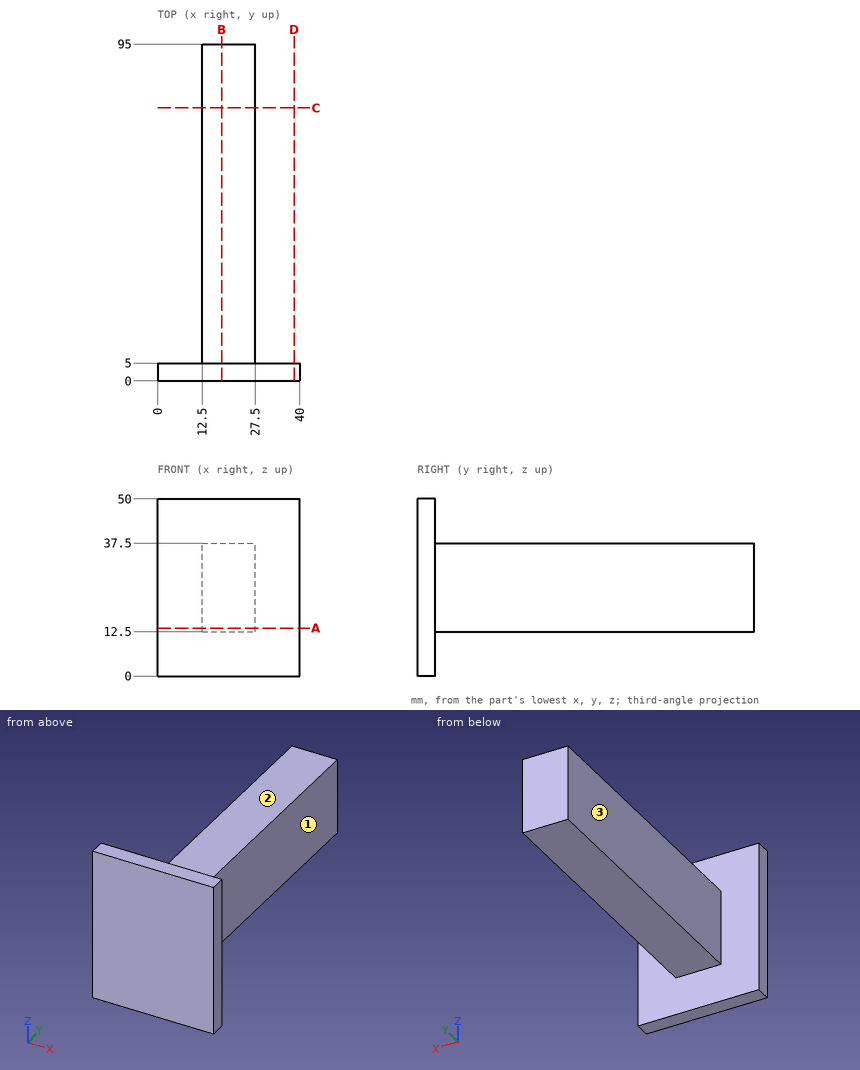
Study the drawing (mm; zero at the part's minimum x, y, z) and answer. A direction names the side the tool comes from. Give positions to 0.01 mm unless a question says otherwise; leave off trailing zeros. Write each loop counter-clockwise with the first axis right and the second up, starting at its lowest first coordinate (ties: lowest second). Pieces come first, ordered by that corner, then holes. Notation, with made-up numbers: (-22, 77) - (-15, 77) arc R11 ccw to (-15, 83) - close; hole circle Ø11 at (80, 68). An arc over 180 degrees is marked (long way). Use a Markdown table: item, result.
1. Section C-C on y = 77 is taken. Write down the section's boundary in (x, z), plus the area to 3 significant figures.
Values follow:
| item | result |
|---|---|
| outline | (12.5, 12.5) - (27.5, 12.5) - (27.5, 37.5) - (12.5, 37.5) - close |
| area | 375 mm² |
2. Section A-A on z = 13.5 is taken. Write down the section's boundary in (x, y), plus the area to 3 significant figures.
Values follow:
| item | result |
|---|---|
| outline | (0, 0) - (40, 0) - (40, 5) - (27.5, 5) - (27.5, 95) - (12.5, 95) - (12.5, 5) - (0, 5) - close |
| area | 1,550 mm² |
3. Each of these flat-tipped pins is pushed along its axis until it touches: P1, Ø12, axis at x = 21.5, y = 48, coming from the +Z side; P2, Ø6, axis at x = 24.5, y = 63.5, coming from the -Z side; P3, Ø2, axis at y = 32, z = 18.5, coming from the -X side. Where does it stop, or does it pass through?
Values follow:
| item | result |
|---|---|
| P1 | stops at z = 37.5 |
| P2 | stops at z = 12.5 |
| P3 | stops at x = 12.5 |
4. A tool of negligible diameter and unlimited length cuts with its end or side. For the marked faces 1, 2 and 3, from which of +Z, -Z, +X, -X, +Y, -Y can it reach the whole face along a straight path? Write none if from no direction.
Values follow:
| item | result |
|---|---|
| face 1 | +Z, -Z, +X, +Y |
| face 2 | +Z, +X, -X, +Y |
| face 3 | +Z, -Z, -X, +Y |
5. Find the intervals of material crossed by probe 1 along Z at (x, y) = (16, 15.5); probe 2 along Y at (x, z) = (30, 38); probe 3 along X at (y, z) = (68.5, 23), in increasing order. Write a range as from..to.
Values follow:
| item | result |
|---|---|
| probe 1 | z = 12.5..37.5 |
| probe 2 | y = 0..5 |
| probe 3 | x = 12.5..27.5 |
6. Section D-D on x = 38.5 is taken. Write down the section's boundary in (y, z), plus the area to 3 significant figures.
Values follow:
| item | result |
|---|---|
| outline | (0, 0) - (5, 0) - (5, 50) - (0, 50) - close |
| area | 250 mm² |
7. Section B-B on x = 18 is taken. Write down the section's boundary in (y, z).
Values follow:
| item | result |
|---|---|
| outline | (0, 0) - (5, 0) - (5, 12.5) - (95, 12.5) - (95, 37.5) - (5, 37.5) - (5, 50) - (0, 50) - close |
